```python
from build123d import *

# Parameters (mm, degrees)
PAD004_DEPTH = 10
SKETCH003_R  = 8.25
PAD003_DEPTH = 10
SKETCH002_W  = 101
SKETCH002_H  = 101
PAD002_DEPTH = 5
SKETCH_W     = 105
SKETCH_H     = 105
PAD_DEPTH    = 5
SKETCH001_W  = 110
SKETCH001_H  = 110
PAD001_DEPTH = 2
CHAMFER_SIZE = 15


with BuildPart() as body003:
    # Sketch004 → Pad004 (new body)
    with BuildSketch(Plane.XY):
        with BuildLine():
            Line((60, -2.5), (60, 2.5))
            Line((60, 2.5), (20, 2.5))
            ThreePointArc((20, 2.5), (17.5, 0), (20, -2.5))
            Line((20, -2.5), (60, -2.5))
        make_face()
    extrude(amount=PAD004_DEPTH)


with BuildPart() as body002:
    # Sketch003 → Pad003 (new body)
    with BuildSketch(Plane.XY):
        with Locations((-23, 0)):
            Circle(SKETCH003_R)
    extrude(amount=PAD003_DEPTH)


with BuildPart() as body001:
    # Sketch002 → Pad002 (new body)
    with BuildSketch(Plane.XY):
        Rectangle(SKETCH002_W, SKETCH002_H)
    extrude(amount=PAD002_DEPTH)


with BuildPart() as chamfer_body:
    # Sketch → Pad (new body)
    with BuildSketch(Plane.XY):
        Rectangle(SKETCH_W, SKETCH_H)
    extrude(amount=PAD_DEPTH)

    # Sketch001 (on Face6 of Pad) → Pad001 (join)
    with BuildSketch(Plane.XY.offset(5)):
        Rectangle(SKETCH001_W, SKETCH001_H)
    extrude(amount=PAD001_DEPTH)

    # Cut: cut Body001
    add(body001.part, mode=Mode.SUBTRACT)

    # Cut001: cut Body002
    add(body002.part, mode=Mode.SUBTRACT)

    # Cut002: cut Body003
    add(body003.part, mode=Mode.SUBTRACT)

    # Chamfer
    chamfer_edges = [chamfer_body.edges().sort_by_distance(p)[0] for p in [
        (-55, 55, 6),
        (55, 55, 6),
        (-55, -55, 6),
        (55, -55, 6),
        (52.5, 52.5, 2.5),
        (-52.5, 52.5, 2.5),
        (-52.5, -52.5, 2.5),
        (52.5, -52.5, 2.5),
        (50.5, 50.5, 2.5),
        (50.5, -50.5, 2.5),
        (-50.5, 50.5, 2.5),
        (-50.5, -50.5, 2.5),
    ]]
    chamfer(chamfer_edges, length=CHAMFER_SIZE)


solid = chamfer_body.part
```
Model file for the job. Use its own axes, mm. A direction names the side the tool comes from. Round coordinates to 2 decimals unless told otherwise and drop trailing zeros. Loops run counter-clockwise (first coordinate to the right, second up) from the corner with the lowest first, then second, coordinate; pieces in that order, holes last. Notation, with made-up numbers: M 79,-37.75 L 102,-37.75 A24 ccw 102,1.25 Z; hole C 68.25,25 d11. An arc over 180 degrees is marked long. Put each result on its own line as item: value. Start each with the question number.
Item 1: Cut at C-C (x = 13). List the corners of the cut face in (y, z), then the cut area to 3 significant figures.
Item 2: Drop flat-ended pins along their axis: P1, Ø1, axis at x = 1, z = 3, coming from the +Y side; P2, Ø4, axis at x = -12, z = 1.5, coming from the -Y side; P3, Ø1.5, axis at y = 42.5, z = 4, coming from the -X side. Give the stop position or say it passes through.
Item 3: Cut at B-B (x = -23). List the corners of the cut face in (y, z).
Item 4: Cut at A-A (y = 0). List the corners of the cut face in (x, z).
Item 5: 3-axis set-ups, long thin cutter, end or side, ignore diameter. For faces 4 (the face through (43, -43, 2)), 5 (the face through (-1, 52.5, 2)), 6 (the face through (38.7, -2.5, 5.3)), 7 (the face through (52.5, 20, 2)), 8 (the face through (45, 45, 2)): which of +Z, -Z, +X, -X, +Y, -Y reach the whole face in a straight line?
Item 6: Cut at D-D (y = -43.5). List the corners of the cut face in (x, z), then the cut area to 3 significant figures.
Item 7: Mould opens along X. For faces 1 (the face through (-51, 20, 0)), 2 (the face through (48, -47, 6)), 3 (the face through (0, 50.5, 2)) say: released by +X, released by -X, zero draft, split by the parting line, or undercut.
Item 8: Drill centre lines: line 1 along Y through (x, z) = (18.5, 2.75); line 2 along X through (y, z) = (0, 6.5); line 3 along Y through (x, z) = (-23, 5.75). Where is each one in solid material? Low to high.
Answer block:
1. outline: M -55,5 L -52.5,5 L -52.5,0 L -50.5,0 L -50.5,5 L 50.5,5 L 50.5,0 L 52.5,0 L 52.5,5 L 55,5 L 55,7 L -55,7 Z
1. area: 240 mm2
2. P1: y = 52.5
2. P2: y = -52.5
2. P3: x = -48.25
3. outline: M -55,5 L -52.5,5 L -52.5,0 L -50.5,0 L -50.5,5 L -8.25,5 L -8.25,7 L -55,7 Z; M 8.25,5 L 50.5,5 L 50.5,0 L 52.5,0 L 52.5,5 L 55,5 L 55,7 L 8.25,7 Z
4. outline: M -55,5 L -52.5,5 L -52.5,0 L -50.5,0 L -50.5,5 L -31.25,5 L -31.25,7 L -55,7 Z; M -14.75,5 L 17.5,5 L 17.5,7 L -14.75,7 Z
5. face 4: -Z
5. face 5: -Z, +X, -X, +Y
5. face 6: +Z, -Z, +X
5. face 7: -Z, +X, +Y, -Y
5. face 8: -Z, +X, +Y
6. outline: M -51.5,5 L -46.5,5 L -46.5,0 L -42.5,0 L -42.5,5 L 42.5,5 L 42.5,0 L 46.5,0 L 46.5,5 L 51.5,5 L 51.5,7 L -51.5,7 Z
6. area: 246 mm2
7. face 1: zero draft
7. face 2: released by +X
7. face 3: undercut
8. line 1: -52.5 to -50.5, 50.5 to 52.5
8. line 2: -55 to -31.25, -14.75 to 17.5
8. line 3: -55 to -8.25, 8.25 to 55
